```python
from build123d import *

# Parameters (mm, degrees)
SKETCH1_R           = 11.9
BOSS_EXTRUDE1_DEPTH = 2
SKETCH2_W           = 1.2
SKETCH2_H           = 1.25
BOSS_EXTRUDE2_DEPTH = 4
SKETCH3_W           = 1.2
SKETCH3_H           = 1.4
BOSS_EXTRUDE3_DEPTH = 2
SKETCH4_W           = 1.2
SKETCH4_H           = 1.4
BOSS_EXTRUDE4_DEPTH = 2


with BuildPart() as part:
    # Sketch1 → Boss-Extrude1 (new body)
    with BuildSketch(Plane.XY):
        Circle(SKETCH1_R)
    extrude(amount=BOSS_EXTRUDE1_DEPTH)

    # Sketch2 → Boss-Extrude2 (add)
    with BuildSketch(Plane.XY.offset(2)):
        with Locations((10.203511987, 1.056286149)):
            Rectangle(SKETCH2_W, SKETCH2_H)
        with Locations((-10.203511987, 1.056286149)):
            Rectangle(SKETCH2_W, SKETCH2_H)
    extrude(amount=BOSS_EXTRUDE2_DEPTH)

    # Sketch3 → Boss-Extrude3 (add)
    with BuildSketch(Plane(origin=(0, 1.681286149, 0), x_dir=(1, 0, 0), z_dir=(0, 1, 0))):
        with Locations((-10.203511987, -5.3)):
            Rectangle(SKETCH3_W, SKETCH3_H)
    extrude(amount=BOSS_EXTRUDE3_DEPTH)

    # Sketch4 → Boss-Extrude4 (add)
    with BuildSketch(Plane.XZ.offset(-0.431286149)):
        with Locations((10.203511987, 5.3)):
            Rectangle(SKETCH4_W, SKETCH4_H)
    extrude(amount=BOSS_EXTRUDE4_DEPTH)


solid = part.part
```
The model under review builds one solid part; all positions refer to its coordinate system, in mm. A direction names the side the tool comes from. Round coordinates to 2 decimals unless told otherwise and drop trailing zeros. Order: outer loops, then holes, each group sorted by start corner. A loop starts at its lowest first (then second) coordinate and runs counter-clockwise, first axis right, second up. Notation, with made-up numbers: (44, 80.25) -> (54, 80.25) arc R18 ccw to (54, 100.25) -> close; hole circle Ø9 at (49, 5.25). An arc over 180 degrees is marked (long way). Use a Markdown table: item, result.
Q1. We need section A-A on z = 5.4. Write out the cut boundary in (x, y), then the cut area to 3 significant figures.
Values:
| item | result |
|---|---|
| outline | (-10.8, 0.43) -> (-9.6, 0.43) -> (-9.6, 3.68) -> (-10.8, 3.68) -> close; (9.6, -1.57) -> (10.8, -1.57) -> (10.8, 1.68) -> (9.6, 1.68) -> close |
| area | 7.80 mm^2 |
Q2. We need section C-C on x = 0. Write out the cut boundary in (y, z), then the cut area to 3 significant figures.
Values:
| item | result |
|---|---|
| outline | (-11.9, 0) -> (11.9, 0) -> (11.9, 2) -> (-11.9, 2) -> close |
| area | 47.6 mm^2 |
Q3. For line 1 (Z direction, x = -6.5, y = -4.25); line 2 (X direction, y = 1, z = 3.95); line 3 (Y direction, x = 0.25, z = 1.65), list the stretches that pass through material, from the lowest coordinate up.
Values:
| item | result |
|---|---|
| line 1 | z = 0 to 2 |
| line 2 | x = -10.8 to -9.6, 9.6 to 10.8 |
| line 3 | y = -11.9 to 11.9 |
Q4. We need section B-B on y = 0. Write out the cut boundary in (x, z).
Values:
| item | result |
|---|---|
| outline | (-11.9, 0) -> (11.9, 0) -> (11.9, 2) -> (-11.9, 2) -> close; (9.6, 4.6) -> (10.8, 4.6) -> (10.8, 6) -> (9.6, 6) -> close |
Q5. We need section D-D on y = 10.5. Write out the cut boundary in (x, z), then the cut area to 3 significant figures.
Values:
| item | result |
|---|---|
| outline | (-5.6, 0) -> (5.6, 0) -> (5.6, 2) -> (-5.6, 2) -> close |
| area | 22.4 mm^2 |
Q6. Tool access review of faces 5 (the flat face through (-10, 3, 4.6)), 6 (the flat face through (10, -1, 4.6)), 7 (the flat face through (-10, 0.431, 4)), 8 (the flat face through (10.804, 1, 4)): name each direction out of +Z, -Z, +X, -X, +Y, -Y from which nothing blocks a thin tool from reaching the whole face with its end or side.
Values:
| item | result |
|---|---|
| face 5 | +X, -X, +Y |
| face 6 | +X, -X, -Y |
| face 7 | +Z, -X, -Y |
| face 8 | +Z, +X, +Y, -Y |
Q7. Mouldability with a two-part tool opening along X and no side actions: class faces 1 (the flat face through (-9.604, 1, 4)), 2 (the flat face through (-10.804, 1, 4)), 3 (the flat face through (10, -1.569, 5)), 4 (the flat face through (9.604, 1, 4)) as +X half, -X half, draft (parallel to the pull), parting line (faces both ways), or undercut.
Values:
| item | result |
|---|---|
| face 1 | undercut |
| face 2 | -X half |
| face 3 | draft |
| face 4 | undercut |
Q8. Clearance check with flat-ended pins moving along their axes: P1, Ø1, axis at x = -10.5, z = 3, coming from the +Y side; P2, Ø1, axis at x = 9, z = 2, coming from the +Y side; P3, Ø2.5, axis at y = 1, z = 4.5, coming from the +X side. State where each tip first meets the part, or that it passes through.
Values:
| item | result |
|---|---|
| P1 | stops at y = 1.68 |
| P2 | stops at y = 8.33 |
| P3 | stops at x = 10.8 |
